Geometry: final body of the model. Coordinates: model frame, mm. Round coordinates to 2 decimals unless told otherwise and drop trailing zeros. Order: outer loops, then holes, each group sorted by start corner. A loop starts at its lowest first (then second) coordinate and runs counter-clockwise, first axis right, second up. Notation, with made-up numbers: M -39.75,6 L -28.75,6 A21 cw -28.75,30 Z; hole C 30,-6 d1. An arc over 180 degrees is marked long. Return JSON: item names as keys, results as strings. Group by question number.
Q1. Cut plane A-A on z = 13. Count the separate pieces of the cut face and the enclosed holes in it, and give its area (3 significant figures).
Q2. Contact query for flat-ended pins moving along their axis: pin 1 (1.4 mm diameter, centred on y = 1.5, z = 14.5, fed in from -X); pin 2 (6 mm diameter, centred on y = 16.5, z = 6, fed in from +X); pin 3 (1 mm diameter, centred on y = 13.5, z = 7, fed in from +X); pin 4 (4 mm diameter, centred on y = -15.5, z = 13, fed in from +X). Output: stop coordinate, or through.
Q3. Cut plane C-C on x = -83. Output: boundary loops of the cut face in (y, z).
Q4. Ray query, probe 1 along Z at (x, y) = (37, -7.5); probe 2 along Y at (x, z) = (12, 9); probe 3 along Y at (x, z) = (-1, 10.5). Return the intervals inside material, ascending.
Q5. Cut plane B-B on y = -12. Output: boundary loops of the cut face in (x, z).
```python
from build123d import *

# Parameters (mm, degrees)
SKETCH_W            = 360
SKETCH_H            = 50
PAD_DEPTH           = 10
PAD_TAPER           = 3
PAD001_DEPTH        = 8
LINEARPATTERN_COUNT = 5
LINEARPATTERN_PITCH = 60


with BuildPart() as part:
    # Sketch → Pad (new body)
    with BuildSketch(Plane.XY):
        Rectangle(SKETCH_W, SKETCH_H)
    extrude(amount=PAD_DEPTH, taper=PAD_TAPER)

    # Sketch001 (on DatumPlane) → Pad001 (join)
    with BuildSketch(Plane.XY.offset(10)):
        Polygon((-120.6, 1.9), (-119.4, 1.9), (-119.4, 0.6), (-118.1, 0.6), (-118.1, -0.6), (-119.4, -0.6), (-119.4, -1.9), (-120.6, -1.9), (-120.6, -0.6), (-121.9, -0.6), (-121.9, 0.6), (-120.6, 0.6), align=None)
    pad001 = extrude(amount=PAD001_DEPTH)

    # LinearPattern: Pad001 ×5
    with Locations(*[(i * LINEARPATTERN_PITCH, 0, 0) for i in range(1, LINEARPATTERN_COUNT)]):
        add(pad001)


solid = part.part
```
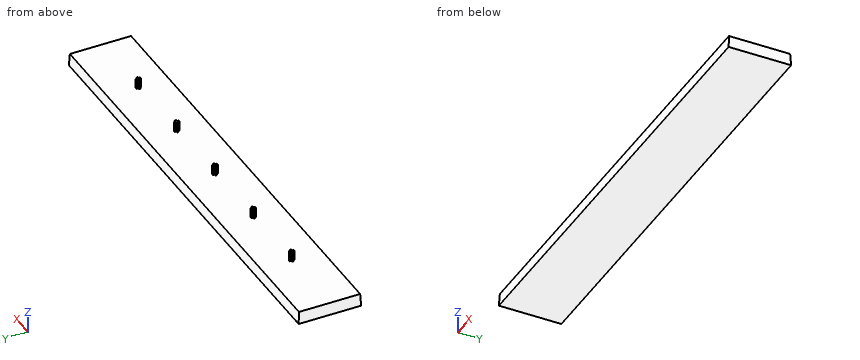
Result sheet:
{
 "1": {"separate pieces": "5", "enclosed holes": "0", "area": "38.4 mm²"},
 "2": {"pin 1": "stops at x = -120.6", "pin 2": "stops at x = 179.84", "pin 3": "stops at x = 179.66", "pin 4": "passes through"},
 "3": {"outline": "M -25,0 L 25,0 L 24.48,10 L -24.48,10 Z"},
 "4": {"probe 1": "z = 0 to 10", "probe 2": "y = -24.53 to 24.53", "probe 3": "y = -0.6 to 0.6"},
 "5": {"outline": "M -180,0 L 180,0 L 179.48,10 L -179.48,10 Z"}
}
